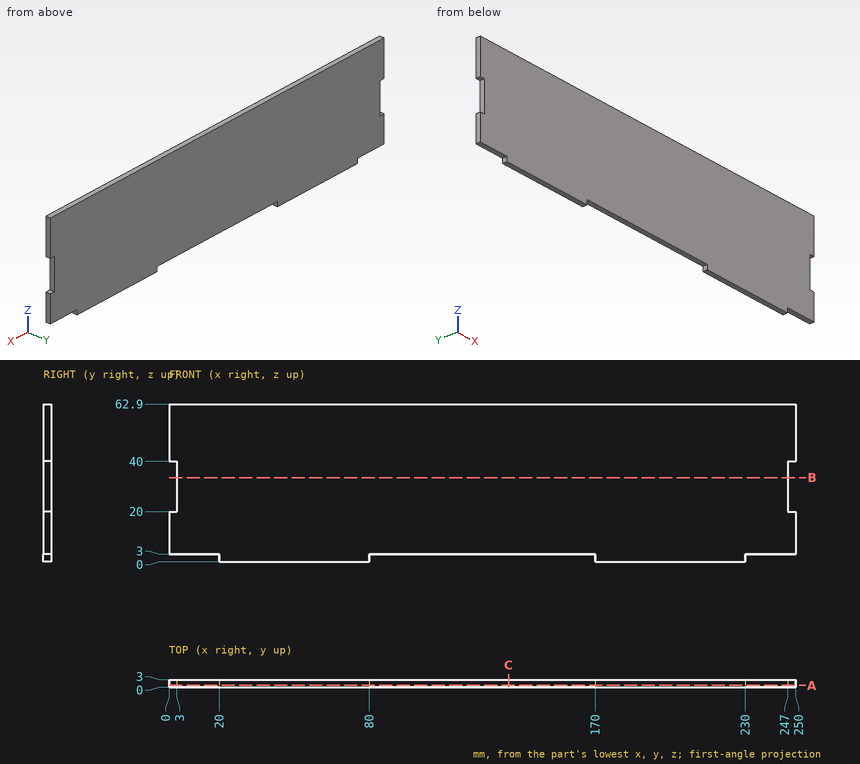
Geometry: see drawing. Coordinates: mm, zero at the bounding-box minimum. Coordinates: 2 decimals unless noted, no trailing zeros. Write each loop counter-clockwise with the first axis right and the second up, starting at its lowest first coordinate (ties: lowest second). Pieces come first, ordered by that corner, then holes. Notation, with made-up numbers: M -18.75,-16.75 L 32.25,-16.75 A18 cw 32.25,2.25 Z; hole C 47,78.25 d11. An arc over 180 degrees is marked long. Use CSV: the item, a comma, the result in double quotes. Start each with the question number.
1. Cut plane A-A on y = 0.7. Return the cut outline in (x, z).
2. First-contact query: P1, Ø0.9, axis at y = 1.5, z = 2, coming from the +X side; P2, Ø1.5, axis at x = 108, y = 1, coming from the -Z side; P3, Ø0.9, axis at y = 1.5, z = 35, coming from the +X side; P4, Ø1.5, axis at y = 1, z = 52.5, coming from the -X side. Flat tips, straight axial feed; report the tip coordinate or a pass-through.
3. Ray query, probe 1 along Z at (x, y) = (139, 1); probe 2 along X at (y, z) = (0.8, 20.5). Return the intervals inside material, ascending.
4. Cut plane C-C on x = 135.5. Return the cut outline in (y, z).
5. Cut plane B-B on z = 33.5. Return the cut outline in (x, y), plus the area to 3 significant figures.
Entries:
1,outline,"M 0,3 L 20,3 L 20,0 L 80,0 L 80,3 L 170,3 L 170,0 L 230,0 L 230,3 L 250,3 L 250,20 L 247,20 L 247,40 L 250,40 L 250,62.9 L 0,62.9 L 0,40 L 3,40 L 3,20 L 0,20 Z"
2,P1,"x = 230"
2,P2,"z = 3"
2,P3,"x = 247"
2,P4,"x = 0"
3,probe 1,"3 to 62.9"
3,probe 2,"3 to 247"
4,outline,"M 0,3 L 3,3 L 3,62.9 L 0,62.9 Z"
5,outline,"M 3,0 L 247,0 L 247,3 L 3,3 Z"
5,area,"732 mm²"
